```python
from build123d import *

# Parameters (mm, degrees)
F0_R     = 81.5
F0_R_2   = 2.55
F0_W     = 30
F0_H     = 3
F0_W_2   = 60
F0_H_2   = 10
F1_DEPTH = 3


# Not quite as in the source:
# - a feature names something its author has since deleted; it is built from what else it names


with BuildPart() as f1:
    # F0 (on Top) → F1 (new body)
    with BuildSketch(Plane.XY):
        Circle(F0_R)
        with Locations((-50, -10)):
            Circle(F0_R_2, mode=Mode.SUBTRACT)
        with Locations((-20, -10)):
            Rectangle(F0_W, F0_H, mode=Mode.SUBTRACT)
        with Locations((20, -10)):
            Rectangle(F0_W, F0_H, mode=Mode.SUBTRACT)
        with Locations((50, -10)):
            Circle(F0_R_2, mode=Mode.SUBTRACT)
        with Locations((-50, 10)):
            Circle(F0_R_2, mode=Mode.SUBTRACT)
        with Locations((-20, 10)):
            Rectangle(F0_W, F0_H, mode=Mode.SUBTRACT)
        Rectangle(F0_W_2, F0_H_2, mode=Mode.SUBTRACT)
        with Locations((20, 10)):
            Rectangle(F0_W, F0_H, mode=Mode.SUBTRACT)
        with Locations((50, 10)):
            Circle(F0_R_2, mode=Mode.SUBTRACT)
    extrude(amount=F1_DEPTH)


solid = f1.part
```
Could you check a few things on this model? Use its own coordinates, in mm. Coordinates: 2 decimals unless noted, no trailing zeros. Write each loop counter-clockwise with the first axis right and the second up, starting at its lowest first coordinate (ties: lowest second). Pieces come first, ordered by that corner, then holes. Notation, with made-up numbers: M -33,19.25 L 23,19.25 A27 cw 23,54.25 Z; hole C 23.25,23 d7. An arc over 180 degrees is marked long. Answer as CSV lines item,"result". Start each with the question number.
1) I want a section at A-A, the plane x = 0. Please give me the cut outline in (y, z).
2) For P1, Ø1.5, axis at y = 10, z = 2, coming from the -X side; P2, Ø4, axis at x = 50, y = 10, coming from the -Z side; P3, Ø0.9, axis at y = 10, z = 2, coming from the +X side; P4, Ø1, axis at y = -25.5, z = 1.5, coming from the +X side, each with a flat end and sliding along its axis, tell me the tip position at first contact or that it passes through.
3) We'd pull the mould along X, two halves only. Please class faces 1 (the cylindrical face through (75.285, -31.215, 1.479)), 2 (the flat face through (-1, -17, 3)), 3 (the cylindrical face through (47.452, 10.112, 1.479)): +X half, -X half, draft (parallel to the pull), parting line (faces both ways), or undercut.
4) I want a section at C-C, the plane y = 0. Please give me the cut outline in (x, z).
5) I want a section at D-D, the plane x = -50. Please give me the cut outline in (y, z), and give its area (3 significant figures).
6) Please list where these lines run through material, in increasing order: line 1 (Y direction, x = -1, z = 0.7); line 2 (Y direction, x = -50, z = 1.65); line 3 (Y direction, x = 12, z = 2.1). Write a range as from..to.
7) I want a section at B-B, the plane z = 0.75. Give the number of separate pieces and of enclosed holes in the cut face, and give its area (3 significant figures).
Data:
1,outline,"M -81.5,0 L -5,0 L -5,3 L -81.5,3 Z; M 5,0 L 81.5,0 L 81.5,3 L 5,3 Z"
2,P1,"stops at x = -80.97"
2,P2,"passes through"
2,P3,"stops at x = 80.94"
2,P4,"stops at x = 77.57"
3,face 1,"parting line"
3,face 2,"draft"
3,face 3,"undercut"
4,outline,"M -81.5,0 L -30,0 L -30,3 L -81.5,3 Z; M 30,0 L 81.5,0 L 81.5,3 L 30,3 Z"
5,outline,"M -64.36,0 L -12.55,0 L -12.55,3 L -64.36,3 Z; M -7.45,0 L 7.45,0 L 7.45,3 L -7.45,3 Z; M 12.55,0 L 64.36,0 L 64.36,3 L 12.55,3 Z"
5,area,"356 mm^2"
6,line 1,"y = -81.49..-5, 5..81.49"
6,line 2,"y = -64.36..-12.55, -7.45..7.45, 12.55..64.36"
6,line 3,"y = -80.61..-11.5, -8.5..-5, 5..8.5, 11.5..80.61"
7,separate pieces,"1"
7,enclosed holes,"9"
7,area,"19,800 mm^2"
